The drawing under review shows one solid part. Ordinate dimensions are in mm from its lowest x, y, z. Give positions to 0.01 mm unless a question says otherwise; leave off trailing zeros. Write each loop counter-clockwise with the first axis right and the second up, starting at its lowest first coordinate (ties: lowest second). Pieces come first, ordered by that corner, then holes.
Q1. For line 1 (X direction, y = 7.5, z = 0.4); line 2 (Y direction, x = 2, z = 0.35) (1 decimal); line 3 (X direction, y = 13.5, z = 0.45), list the stretches that pass through material, from the lowest coordinate up.
Q2. We need section C-C (x = 10.5). Write out the cut boundary in (y, z).
Q3. We need section A-A (z = 0.25). Give the number of separate pieces and of enclosed holes in the cut face.
Q4. We need section B-B (y = 11.5). Write out the cut boundary in (x, z).
Q5. We need section D-D (y = 8.25). Write out the cut boundary in (x, z).
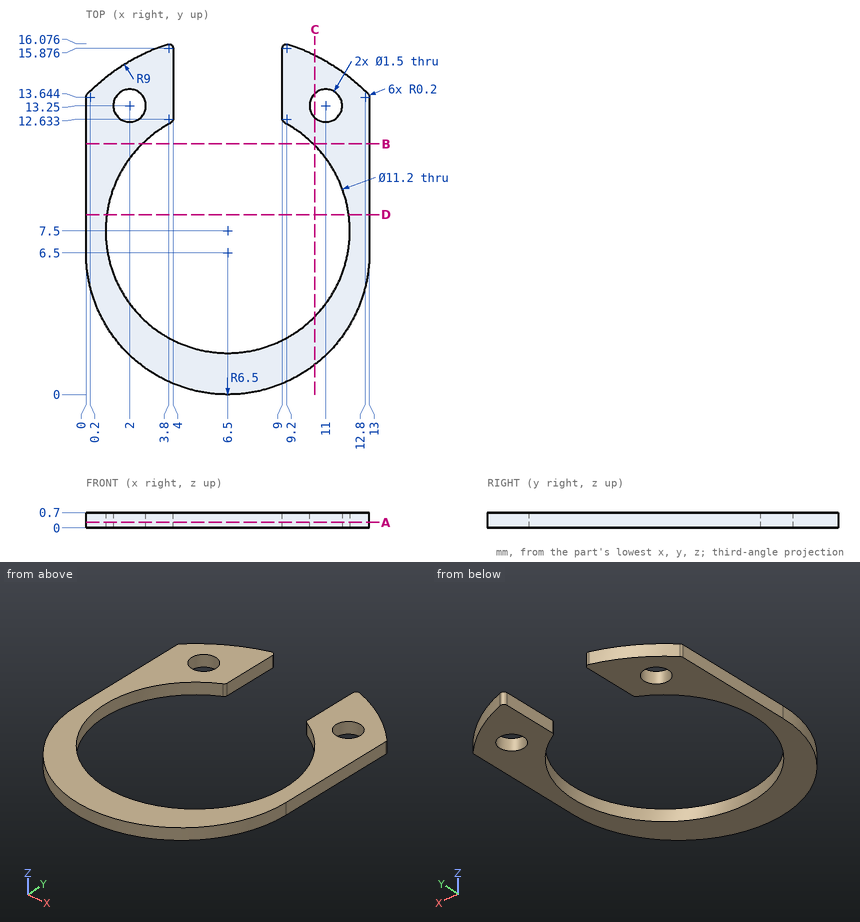
Computed:
1. line 1: x = 0 to 0.9, 12.1 to 13
1. line 2: y = 1.8 to 4.2, 10.8 to 12.5, 14 to 15.3
1. line 3: x = 0 to 1.29, 2.71 to 4, 9 to 10.29, 11.71 to 13
2. outline: (1.38, 0) - (3.58, 0) - (3.58, 0.7) - (1.38, 0.7) - close; (11.42, 0) - (12.69, 0) - (12.69, 0.7) - (11.42, 0.7) - close; (13.81, 0) - (15.56, 0) - (15.56, 0.7) - (13.81, 0.7) - close
3. separate pieces: 1
3. enclosed holes: 2
4. outline: (0, 0) - (2.58, 0) - (2.58, 0.7) - (0, 0.7) - close; (10.42, 0) - (13, 0) - (13, 0.7) - (10.42, 0.7) - close
5. outline: (0, 0) - (0.95, 0) - (0.95, 0.7) - (0, 0.7) - close; (12.05, 0) - (13, 0) - (13, 0.7) - (12.05, 0.7) - close
